Design review of the part built by this model. Coordinates are the model's own, in mm. A direction names the side the tool comes from. Coordinates: 2 decimals unless noted, no trailing zeros. Write each loop counter-clockwise with the first axis right and the second up, starting at its lowest first coordinate (ties: lowest second). Pieces come first, ordered by that corner, then holes.
Q1. Take a section at C-C (z = 16.51). Give the boundary of the cut face in (x, y), and give its area (3 significant figures).
Q2. Machinability: for faces 5 (the flat face through (19.05, -1, 13)), 6 (the flat face through (-8, -38.1, 27)), 7 (the flat face through (-19.05, -1, 13)), which of the approach directions +Z, -Z, +X, -X, +Y, -Y give a long, thin tool a straight path to every point of the face, cutting with its end or side? Answer none if there is none.
Q3. Take a section at B-B (y = -2.5). Give the boundary of the cut face in (x, z), and give its area (3 significant figures).
Q4. Mouldability with a two-part tool opening along Z and no side actions: class faces 1 (the flat face through (-8, 38.1, 27)), 2 (the flat face through (-25, -1, 26.67)), 3 (the flat face through (0, 1, 33.02)), 4 (the cylindrical face through (-1.579, -0.533, 28.535)) as pulls with the +Z half, pulls with the -Z half, needs draft (parallel to the pull), parting line crosses it, or undercut.
Q5. Take a section at D-D (x = -20). Give the boundary of the cut face in (y, z).
Q6. Take a section at A-A (x = 0). Give the boundary of the cut face in (y, z), and give its area (3 significant figures).
Q7. For probe 1 along Z at (x, y) = (0, 0); probe 2 along X at (y, z) = (-17, 16.5); probe 3 along X at (y, z) = (-5.5, 3), list the stretches that pass through material, from the lowest coordinate up.
Q8. Insertion check: pin 1 (5 mm diameter, centred on y = 15, z = 22.5, fed in from +X); pin 2 (4 mm diameter, centred on x = -27, y = -17.5, fed in from -Z); pin 3 (4 mm diameter, centred on y = 18, z = 12.5, fed in from -X). Each pin has a flat end and moves straight along its axis. Give the tip position at first contact, or say it passes through.
```python
from build123d import *

# Parameters (mm, degrees)
F0_W     = 63.5
F0_H     = 76.2
F1_DEPTH = 33.02
F2_R     = 12.1285
F3_DEPTH = 100.076
F4_W     = 12.7
F4_H     = 26.67
F5_DEPTH = 76.201


# Not quite as in the source:
# - a feature names something its author has since deleted; it is built from what else it names


with BuildPart() as f1:
    # F0 (on Top) → F1 (new body)
    with BuildSketch(Plane.XY):
        Rectangle(F0_W, F0_H)
    extrude(amount=F1_DEPTH)

    # F2 (on face) → F3 (cut)
    with BuildSketch(Plane.XZ.offset(38.1)):
        with Locations((0, 16.51)):
            Circle(F2_R)
    extrude(amount=-F3_DEPTH, mode=Mode.SUBTRACT)

    # F4 (on face) → F5 (cut, through all)
    with BuildSketch(Plane.XZ.offset(38.1)):
        with Locations((25.4, 13.335)):
            Rectangle(F4_W, F4_H)
        with Locations((-25.4, 13.335)):
            Rectangle(F4_W, F4_H)
    extrude(amount=-F5_DEPTH, mode=Mode.SUBTRACT)


solid = f1.part
```
Response:
1. outline: (-19.05, -38.1) - (-12.13, -38.1) - (-12.13, 38.1) - (-19.05, 38.1) - close; (12.13, -38.1) - (19.05, -38.1) - (19.05, 38.1) - (12.13, 38.1) - close
1. area: 1,050 mm2
2. face 5: -Z, +X, +Y, -Y
2. face 6: +Z, -Z, +X, -X, -Y
2. face 7: -Z, -X, +Y, -Y
3. outline: (-31.75, 26.67) - (-19.05, 26.67) - (-19.05, 0) - (19.05, 0) - (19.05, 26.67) - (31.75, 26.67) - (31.75, 33.02) - (-31.75, 33.02) - close; hole circle Ø24.26 at (0, 16.51)
3. area: 957 mm2
4. face 1: needs draft
4. face 2: pulls with the -Z half
4. face 3: pulls with the +Z half
4. face 4: undercut
5. outline: (-38.1, 26.67) - (38.1, 26.67) - (38.1, 33.02) - (-38.1, 33.02) - close
6. outline: (-38.1, 0) - (38.1, 0) - (38.1, 4.38) - (-38.1, 4.38) - close; (-38.1, 28.64) - (38.1, 28.64) - (38.1, 33.02) - (-38.1, 33.02) - close
6. area: 668 mm2
7. probe 1: z = 0 to 4.38, 28.64 to 33.02
7. probe 2: x = -19.05 to -12.13, 12.13 to 19.05
7. probe 3: x = -19.05 to 19.05
8. pin 1: stops at x = 19.05
8. pin 2: stops at z = 26.67
8. pin 3: stops at x = -19.05
